Input: part model. Units: mm. Frame: model coordinates. A direction names the side the tool comes from. Coordinates: 2 decimals unless noted, no trailing zeros. Write each loop counter-clockwise with the first axis right and the second up, starting at its lowest first coordinate (ties: lowest second). Pieces come first, ordered by that corner, then holes. Notation, with made-up numbers: (76, 41.5) - (135, 41.5) arc R19 ccw to (135, 45.5) - close; hole circle Ø7 at (-7, 85). An arc over 180 degrees is marked (long way). Use a Markdown table: item, result. Add a question column.
Q1. Section query A-A (x = -123). Return the cut outline in (y, z), then the cut area to 3 significant figures.
Q2. Set-up query: faces 1 (the face through (-147, -44.798, 100)), 2 (the face through (-88.004, -40, 159)), 3 (the face through (25.268, 142, 105)). Return all of +Z, -Z, +X, -X, +Y, -Y with unobstructed straight access to the full face (end or side cutting, diameter ignored); none if empty.
Q3. Mould query, pull axis X, two halves, no side actions, for faces 4 (the face through (-146, -37, 202)), 5 (the face through (-325.412, 151, 100)), 6 (the face through (-313.232, -29.962, 104.656)), 7 (the face through (20.2, 310.6, 104.7)). Classes: released by +X, released by -X, zero draft, split by the parting line, or undercut.
Q4. Section query C-C (z = 160.5). Return the cut outline in (x, y), then the cut area to 3 significant figures.
Q5. Section query D-D (y = 264.5). Return the cut outline in (x, z).
Q6. Material intervals for probe 1 along X at (y, z) = (3, 25.5); probe 2 along Y at (x, z) = (-195, 138); probe 3 along Z at (x, y) = (-96.5, 200.5), sorted ascending. Write a range as from..to.
Q7. Pin query (flat end, axial travel): P1, Ø4, axis at x = 39.5, z = 149, coming from the +Y side; P2, Ø2.5, axis at x = 29, z = 68, coming from the -Y side; P3, Ø4, axis at y = 243, z = 79.5, coming from the +X side; P4, Ø8, axis at x = -172, y = -40, coming from the -Z side. Return the tip coordinate at first contact, or that it passes through.
Q8. Section query B-B (z = 119.5). Return the cut outline in (x, y), then the cut area to 3 significant figures.
from build123d import *

# Parameters (mm, degrees)
BOSS_EXTRUDE1_DEPTH = 10
BOSS_EXTRUDE2_DEPTH = 192
CUT_EXTRUDE1_DEPTH  = 192


with BuildPart() as part:
    # Sketch1 → Boss-Extrude1 (new body)
    with BuildSketch(Plane.XY):
        with BuildLine():
            Line((-325.411527203, 298.102478214), (-325.411527203, 0))
            Line((-325.411527203, 0), (-333.392551687, 0))
            Line((-333.392551687, 0), (-333.392551687, -19.397521786))
            ThreePointArc((-333.392551687, -19.397521786), (-319.468572459, -37.806041519), (-297.471527203, -44.797521786))
            Line((-297.471527203, -44.797521786), (7.328472797, -44.797521786))
            ThreePointArc((7.328472797, -44.797521786), (29.426688427, -37.734255924), (43.331435707, -19.163341521))
            Line((43.331435707, -19.163341521), (43.331435707, 0))
            Line((43.331435707, 0), (35.268472797, 0))
            Line((35.268472797, 0), (35.268472797, 298.102478214))
            ThreePointArc((35.268472797, 298.102478214), (27.085036263, 317.859041681), (7.328472797, 326.042478214))
            Line((7.328472797, 326.042478214), (-297.471527203, 326.042478214))
            ThreePointArc((-297.471527203, 326.042478214), (-317.22809067, 317.859041681), (-325.411527203, 298.102478214))
        make_face()
    extrude(amount=BOSS_EXTRUDE1_DEPTH)

    # Sketch2 → Boss-Extrude2 (add)
    with BuildSketch(Plane.XY.offset(10)):
        with BuildLine():
            Line((-325.411527203, 298.102478214), (-325.411527203, 0))
            Line((-325.411527203, 0), (-333.392551687, 0))
            Line((-333.392551687, 0), (-333.392551687, -19.397521786))
            ThreePointArc((-333.392551687, -19.397521786), (-319.468572459, -37.806041519), (-297.471527203, -44.797521786))
            Line((-297.471527203, -44.797521786), (7.328472797, -44.797521786))
            ThreePointArc((7.328472797, -44.797521786), (29.426688427, -37.734255924), (43.331435707, -19.163341521))
            Line((43.331435707, -19.163341521), (43.331435707, 0))
            Line((43.331435707, 0), (35.268472797, 0))
            Line((35.268472797, 0), (35.268472797, 298.102478214))
            ThreePointArc((35.268472797, 298.102478214), (27.085036263, 317.859041681), (7.328472797, 326.042478214))
            Line((7.328472797, 326.042478214), (-297.471527203, 326.042478214))
            ThreePointArc((-297.471527203, 326.042478214), (-317.22809067, 317.859041681), (-325.411527203, 298.102478214))
        make_face()
        with BuildLine():
            Line((-315.411527203, 298.102478214), (-315.411527203, -10))
            Line((-315.411527203, -10), (-323.392551687, -10))
            Line((-323.392551687, -10), (-323.392551687, -17.546968301))
            ThreePointArc((-323.392551687, -17.546968301), (-313.039772977, -30.090677271), (-297.471527203, -34.797521786))
            Line((-297.471527203, -34.797521786), (7.328472797, -34.797521786))
            ThreePointArc((7.328472797, -34.797521786), (22.985754076, -30.031178656), (33.331435707, -17.349090679))
            Line((33.331435707, -17.349090679), (33.331435707, -10))
            Line((33.331435707, -10), (25.268472797, -10))
            Line((25.268472797, -10), (25.268472797, 298.102478214))
            ThreePointArc((25.268472797, 298.102478214), (20.013968451, 310.787973869), (7.328472797, 316.042478214))
            Line((7.328472797, 316.042478214), (-297.471527203, 316.042478214))
            ThreePointArc((-297.471527203, 316.042478214), (-310.157022858, 310.787973869), (-315.411527203, 298.102478214))
        make_face(mode=Mode.SUBTRACT)
    extrude(amount=BOSS_EXTRUDE2_DEPTH)

    # Sketch3 → Cut-Extrude1 (cut)
    with BuildSketch(Plane.XZ.offset(44.797521786)):
        with BuildLine():
            ThreePointArc((-130.445711932, 167.470752043), (-145.071527203, 175.87248582), (-159.697342474, 167.470752043))
            Line((-159.697342474, 167.470752043), (-130.445711932, 167.470752043))
        make_face()
        with BuildLine():
            ThreePointArc((-159.697342474, 167.470752043), (-162.002770822, 158.941242201), (-159.697342474, 150.411732359))
            Line((-159.697342474, 150.411732359), (-130.445711932, 150.411732359))
            ThreePointArc((-130.445711932, 150.411732359), (-128.72679943, 154.523450388), (-128.140283584, 158.941242201))
            ThreePointArc((-128.140283584, 158.941242201), (-128.72679943, 163.359034014), (-130.445711932, 167.470752043))
            Line((-130.445711932, 167.470752043), (-159.697342474, 167.470752043))
        make_face()
        with BuildLine():
            ThreePointArc((-128.140283584, 158.941242201), (-128.72679943, 154.523450388), (-130.445711932, 150.411732359))
            Line((-130.445711932, 150.411732359), (-88.003795491, 150.411732359))
            Line((-88.003795491, 150.411732359), (-88.003795491, 167.470752043))
            Line((-88.003795491, 167.470752043), (-130.445711932, 167.470752043))
            ThreePointArc((-130.445711932, 167.470752043), (-128.72679943, 163.359034014), (-128.140283584, 158.941242201))
        make_face()
        with BuildLine():
            Line((-202.139258915, 167.470752043), (-202.139258915, 150.411732359))
            Line((-202.139258915, 150.411732359), (-159.697342474, 150.411732359))
            ThreePointArc((-159.697342474, 150.411732359), (-162.002770822, 158.941242201), (-159.697342474, 167.470752043))
            Line((-159.697342474, 167.470752043), (-202.139258915, 167.470752043))
        make_face()
        with BuildLine():
            Line((-130.445711932, 150.411732359), (-159.697342474, 150.411732359))
            ThreePointArc((-159.697342474, 150.411732359), (-145.071527203, 142.009998582), (-130.445711932, 150.411732359))
        make_face()
    extrude(amount=-CUT_EXTRUDE1_DEPTH, mode=Mode.SUBTRACT)


solid = part.part
Values follow:
| question | item | result |
|---|---|---|
| 1 | outline | (-44.8, 0) - (326.04, 0) - (326.04, 202) - (316.04, 202) - (316.04, 10) - (-34.8, 10) - (-34.8, 150.41) - (-44.8, 150.41) - close; (-44.8, 167.47) - (-34.8, 167.47) - (-34.8, 202) - (-44.8, 202) - close |
| 1 | area | 7,380 mm2 |
| 2 | face 1 | +Z, -Z, +X, -X, -Y |
| 2 | face 2 | -Y |
| 2 | face 3 | +Z |
| 3 | face 4 | zero draft |
| 3 | face 5 | released by -X |
| 3 | face 6 | undercut |
| 3 | face 7 | undercut |
| 4 | outline | (-333.39, -19.4) arc R38.1 ccw to (-297.47, -44.8) - (-202.14, -44.8) - (-202.14, -34.8) - (-297.47, -34.8) arc R28.1 cw to (-323.39, -17.55) - (-323.39, -10) - (-315.41, -10) - (-315.41, 298.1) arc R17.94 cw to (-297.47, 316.04) - (7.33, 316.04) arc R17.94 cw to (25.27, 298.1) - (25.27, -10) - (33.33, -10) - (33.33, -17.35) arc R28.1 cw to (7.33, -34.8) - (-88, -34.8) - (-88, -44.8) - (7.33, -44.8) arc R38.1 ccw to (43.33, -19.16) - (43.33, 0) - (35.27, 0) - (35.27, 298.1) arc R27.94 ccw to (7.33, 326.04) - (-297.47, 326.04) arc R27.94 ccw to (-325.41, 298.1) - (-325.41, 0) - (-333.39, 0) - close |
| 4 | area | 13,000 mm2 |
| 5 | outline | (-325.41, 0) - (35.27, 0) - (35.27, 202) - (25.27, 202) - (25.27, 10) - (-315.41, 10) - (-315.41, 202) - (-325.41, 202) - close |
| 6 | probe 1 | -325.41..-315.41, 25.27..35.27 |
| 6 | probe 2 | -44.8..-34.8, 316.04..326.04 |
| 6 | probe 3 | 0..10 |
| 7 | P1 | y = 0 |
| 7 | P2 | y = -38.86 |
| 7 | P3 | x = 35.27 |
| 7 | P4 | z = 0 |
| 8 | outline | (-333.39, -19.4) arc R38.1 ccw to (-297.47, -44.8) - (7.33, -44.8) arc R38.1 ccw to (43.33, -19.16) - (43.33, 0) - (35.27, 0) - (35.27, 298.1) arc R27.94 ccw to (7.33, 326.04) - (-297.47, 326.04) arc R27.94 ccw to (-325.41, 298.1) - (-325.41, 0) - (-333.39, 0) - close; hole (-323.39, -17.55) arc R28.1 ccw to (-297.47, -34.8) - (7.33, -34.8) arc R28.1 ccw to (33.33, -17.35) - (33.33, -10) - (25.27, -10) - (25.27, 298.1) arc R17.94 ccw to (7.33, 316.04) - (-297.47, 316.04) arc R17.94 ccw to (-315.41, 298.1) - (-315.41, -10) - (-323.39, -10) - close |
| 8 | area | 14,100 mm2 |
